from build123d import *

# Parameters (mm, degrees)
ESBO_O3_W                = 1.1
ESBO_O3_H                = 7.097813332
CORTE_EXTRUS_O1_DEPTH    = 2
ESBO_O4_R                = 1
RESSALTO_EXTRUS_O1_DEPTH = 2
ESBO_O8_R                = 1
CORTE_EXTRUS_O2_DEPTH    = 2
CHANFRO2_SIZE            = 3.4
CHANFRO2_SIZE2           = 1.962990915
CHANFRO3_SIZE            = 0.3


with BuildPart() as part:
    # Esboço1 → Revolução1 (revolve)
    with BuildSketch(Plane(origin=(0, 0, 0), x_dir=(1, 0, 0), z_dir=(0, 1, 0)), mode=Mode.PRIVATE) as revolu_o1_sk:
        Polygon((0, 0), (32, 0), (32, 3), (2, 3), (2, 5), (0, 5), align=None)
    revolve(revolu_o1_sk.sketch.rotate(Axis((0, 0, 0), (1, 0, 0)), 180), axis=Axis((0, 0, 0), (1, 0, 0)))

    # Esboço3 → Corte-extrusão1 (cut)
    with BuildSketch(Plane(origin=(32, 0, 0), x_dir=(0, 0, -1), z_dir=(1, 0, 0))):
        with Locations((0, 0.230257265)):
            Rectangle(ESBO_O3_W, ESBO_O3_H)
    extrude(amount=-CORTE_EXTRUS_O1_DEPTH, mode=Mode.SUBTRACT)


with BuildPart() as body_2:
    # Esboço4 → Ressalto-extrusão1 (new body)
    with BuildSketch(Plane.ZY):
        Circle(ESBO_O4_R)
    extrude(amount=-RESSALTO_EXTRUS_O1_DEPTH)


with BuildPart() as corte_extrus_o2_tool:
    # Esboço8 → Corte-extrusão2 (new body)
    with BuildSketch(Plane.ZY):
        Circle(ESBO_O8_R)
    extrude(amount=-CORTE_EXTRUS_O2_DEPTH)


with BuildPart() as part_1:
    add(part.part)

    # Corte-extrusão2: cut by corte_extrus_o2_tool
    add(corte_extrus_o2_tool.part, mode=Mode.SUBTRACT)

    # Chanfro2
    chanfro2_edges = [part_1.edges().sort_by_distance(p)[0] for p in [
        (0, 0, -1),
    ]]
    chanfro2_side = [part_1.faces().sort_by_distance(p)[0] for p in [
        (0, 0, -4.858578644),
    ]]
    chamfer(chanfro2_edges, length=CHANFRO2_SIZE, length2=CHANFRO2_SIZE2, reference=chanfro2_side[0])

    # Chanfro3
    chanfro3_edges = [part_1.edges().sort_by_distance(p)[0] for p in [
        (0, 0, -5),
        (2, 0, -5),
    ]]
    chamfer(chanfro3_edges, length=CHANFRO3_SIZE)


with BuildPart() as body_2_1:
    add(body_2.part)

    # Corte-extrusão2: cut by corte_extrus_o2_tool
    add(corte_extrus_o2_tool.part, mode=Mode.SUBTRACT)


solid = part_1.part
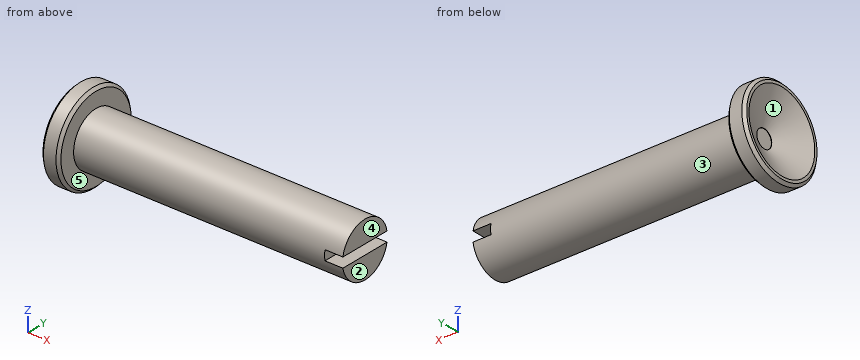
Verification items for the finished model (mm, model axes). Face numbers are marked on the shaded views. A direction names the side the tool comes from. Coordinates: 2 decimals unless noted, no trailing zeros. Order: outer loops, then holes, each group sorted by start corner. A loop starts at its lowest first (then second) coordinate and runs counter-clockwise, first axis right, second up.
1. Release check for a two-part mould opening along Z. For the marked faces 1, 2 and 3 record: +Z half, -Z half, draft (parallel to the pull), parting line (faces both ways), or undercut.
Results found:
face 1: undercut
face 2: draft
face 3: parting line
2. Sectioned sample at C-C, the plane x = 19. Record the cut outline in (y, z).
Results found:
outline: circle Ø6 at (0, 0)
3. Go/stop test with flat-tipped pins: pin 1 Ø2.5 at (y, z) = (0, 0) entering from -X; pin 2 Ø1 at (x, z) = (18, -2.5) entering from -Y; pin 3 Ø0.9 at (y, z) = (-1, 0) entering from +X. Record where each tip stops, or that it passes through.
Results found:
pin 1: stops at x = 1.82
pin 2: stops at y = -2.24
pin 3: stops at x = 30
4. Set-up check for the marked faces 4 and 5: record each of +Z, -Z, +X, -X, +Y, -Y from which the full face is reachable in a straight line by a thin tool's end or side.
Results found:
face 4: +Z, -Z, +X, +Y, -Y
face 5: +X
5. Scan lines: line 1 (X direction, y = 1, z = 4.5); line 2 (X direction, y = 2, z = -1.75); line 3 (Y direction, x = 2.05, z = 0). Record each from-to range of solid material in increasing order.
Results found:
line 1: x = 0 to 2
line 2: x = 1.01 to 32
line 3: y = -3 to 3
